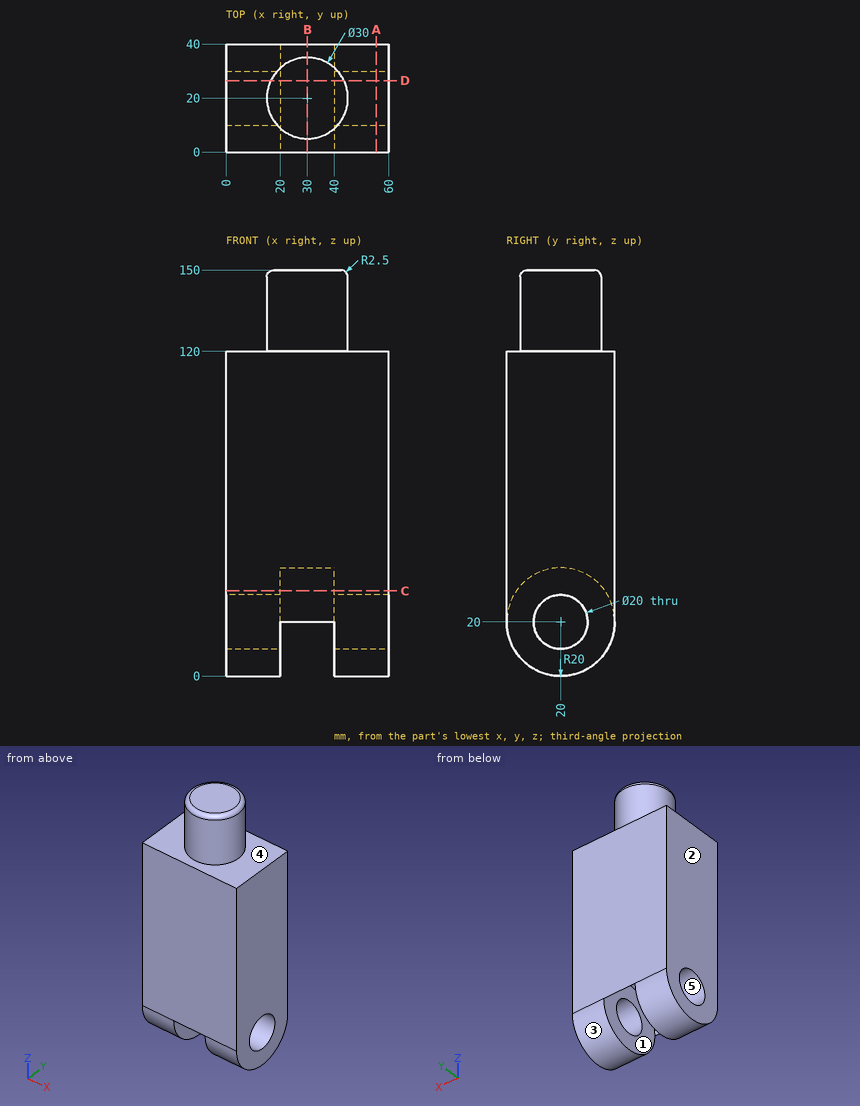
Study the drawing (mm; zero at the part's minimum x, y, z) and answer. A direction names the side the tool comes from. Coordinates: 2 decimals unless noted, no trailing zeros. Write each loop counter-clockwise with the first axis right and the second up, starting at its lowest first coordinate (ties: lowest second). Pieces come first, ordered by that corner, then holes. Notation, with made-up numbers: (78, -39.75) - (115, -39.75) arc R22 ccw to (115, -1.75) - close; hole circle Ø3 at (14, 43). An arc over 180 degrees is marked (long way). Answer as a JSON object with one key per item and string values.
Q1. For a pull along Y with two mould halves and no side action, classify the marked faces 1, 2 and 3 as pulls with the +Y half, pulls with the -Y half, needs draft (parallel to the pull), parting line crosses it, or undercut.
Results list:
{"face 1": "undercut", "face 2": "needs draft", "face 3": "parting line crosses it"}
Q2. Find section C-C (z = 31.5). Write down the section's boundary in (x, y), plus the area to 3 significant figures.
Results list:
{"outline": "(0, 0) - (60, 0) - (60, 40) - (0, 40) - close; hole (20, 3.64) - (40, 3.64) - (40, 36.36) - (20, 36.36) - close", "area": "1,750 mm^2"}
Q3. Which of the six approach directions +Z, -Z, +X, -X, +Y, -Y give full straight-line access (tool end or side, diameter ignored) to the marked faces 4 and 5?
Results list:
{"face 4": "+Z", "face 5": "+X, -X"}
Q4. Find section D-D (y = 26.5). State how many separate pieces and enclosed holes the cut face has, plus the area to 3 significant figures.
Results list:
{"separate pieces": "3", "enclosed holes": "0", "area": "6,580 mm^2"}
Q5. Given pin 1 Ø2 at (x, y) = (35.5, 7.5) entering from -Z; pin 2 Ø8 at (x, z) = (33.5, 35) entering from -Y, each flat-ended and moving along its own axis, determine where each tip first touches the part or whether it passes through.
Results list:
{"pin 1": "stops at z = 34.76", "pin 2": "stops at y = 0"}
Q6. Consider L1, parallel to X at y = 8, z = 34.5; L2, parallel to Z at x = 51, y = 20; L3, parallel to Y at x = 13.5, z = 20. Determine where each line is inside the solid, lowest interval first. Write a range as from..to.
Results list:
{"L1": "x = 0..20, 40..60", "L2": "z = 0..10, 30..120", "L3": "y = 0..10, 30..40"}
Q7. Find section B-B (x = 30). Write down the section's boundary in (y, z).
Results list:
{"outline": "(0, 20) arc R20 cw to (40, 20) - (40, 120) - (35, 120) - (35, 147.5) arc R2.5 ccw to (32.5, 150) - (7.5, 150) arc R2.5 ccw to (5, 147.5) - (5, 120) - (0, 120) - close"}
Q8. Find section A-A (x = 55.5). Write down the section's boundary in (y, z).
Results list:
{"outline": "(0, 20) arc R20 ccw to (40, 20) - (40, 120) - (0, 120) - close; hole circle Ø20 at (20, 20)"}
